from build123d import *

# Parameters (mm, degrees)
SKETCH_W      = 800
SKETCH_H      = 500
PAD_DEPTH     = 750
SKETCH001_W   = 816.672542
SKETCH001_H   = 515.040198
PAD001_DEPTH  = 50
SKETCH002_W   = 715.631729
SKETCH002_H   = 638.12648
POCKET_DEPTH  = 20
SKETCH003_R   = 15.413666
SKETCH003_R_2 = 14.535816
PAD002_DEPTH  = 10
SKETCH004_W   = 32.008468
SKETCH004_H   = 201.831192
PAD003_DEPTH  = 10


with BuildPart() as part:
    # Sketch → Pad (new body)
    with BuildSketch(Plane.XZ):
        with Locations((400, 250)):
            Rectangle(SKETCH_W, SKETCH_H)
    extrude(amount=PAD_DEPTH)

    # Sketch001 (on Face5 of Pad) → Pad001 (join)
    with BuildSketch(Plane(origin=(0, 0, 0), x_dir=(1, 0, 0), z_dir=(0, 1, 0))):
        with Locations((397.221163, -247.606335)):
            Rectangle(SKETCH001_W, SKETCH001_H)
    extrude(amount=-PAD001_DEPTH)

    # Sketch002 (on Face6 of Pad001) → Pocket (cut)
    with BuildSketch(Plane(origin=(0, 0, 0), x_dir=(1, 0, 0), z_dir=(0, 0, -1))):
        with Locations((402.8294, 386.143486)):
            Rectangle(SKETCH002_W, SKETCH002_H)
    extrude(amount=-POCKET_DEPTH, mode=Mode.SUBTRACT)

    # Sketch003 (on Face16 of Pocket) → Pad002 (join)
    with BuildSketch(Plane(origin=(0, 0, 20), x_dir=(1, 0, 0), z_dir=(0, 0, -1))):
        with Locations((80.433578, 384.418488)):
            Circle(SKETCH003_R)
        with Locations((79.198502, 264.994965)):
            Circle(SKETCH003_R_2)
    extrude(amount=PAD002_DEPTH)

    # Sketch004 (on Face20 of Pad002) → Pad003 (join)
    with BuildSketch(Plane(origin=(0, 0, 10), x_dir=(1, 0, 0), z_dir=(0, 0, -1))):
        with Locations((80.688408, 324.975487)):
            Rectangle(SKETCH004_W, SKETCH004_H)
    extrude(amount=PAD003_DEPTH)


solid = part.part
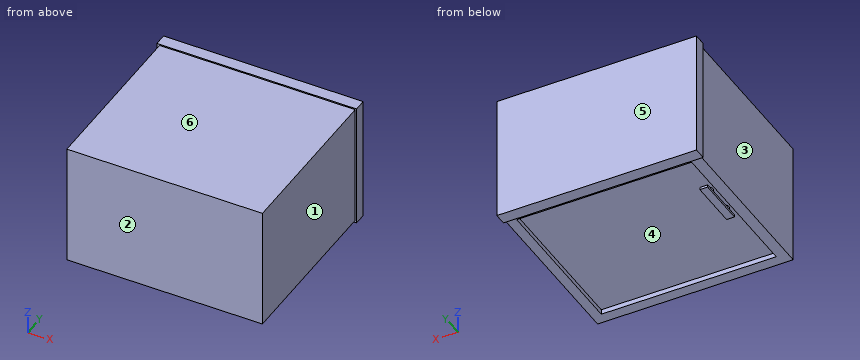
Here's how the part is built. I have some questions about the finished solid (model axes, mm). Face numbers are marked on the shaded views. A direction names the side the tool comes from. Round coordinates to 2 decimals unless told otherwise and drop trailing zeros. Loops run counter-clockwise (first coordinate to the right, second up) from the corner with the lowest first, then second, coordinate; pieces in that order, holes last. Notation, with made-up numbers: M -11,5.25 L 48,5.25 A31 ccw 48,29.25 Z; hole C 64,66.5 d1. An arc over 180 degrees is marked long. Write each question's results on one line, items separated by ' | '. Start each with the question number.
(1) On a 3-axis mill with a long thin cutter (end or side, diameter ignored), from which of +Z, -Z, +X, -X, +Y, -Y can I reach the whole of each face in a straight line? I mean the marked faces 1, 2 and 3. Say none if no direction works.
(2) Will these pins go through, and if not, where does the flat tip stop? P1, Ø2, axis at x = 563.5, y = -77, coming from the +Z side; P2, Ø5, axis at y = -286, z = 4.5, coming from the +X side; P3, Ø22, axis at y = -416.5, z = 10.5, coming from the -X side.
(3) Thinking about a two-plate mould opening in Y: for the marked faces 4, 5 and 6, which applies, pulls with the +Y half, pulls with the -Y half, needs draft (parallel to the pull), parting line crosses it, or undercut?
(4) I want a section at A-A (x = 120). Please give me the cut outline in (y, z), then the cut area to 3 significant figures.
(5) I want a section at C-C (y = -191.5). Please give me the cut outline in (x, z), then the cut area to 3 significant figures.
(6) I want a section at B-B (z = 350). Please give me the cut outline in (x, y).
(7) If I drill on probe 1 along X at (y, z) = (-676.5, 15); probe 2 along X at (y, z) = (-493.5, 214.5); probe 3 along Z at (x, y) = (150, -135.5), over which ranges is the centre line in solid material (lowest first)? Write a range as from..to.
Solved:
1) face 1: +Z, -Z, +X, -Y | face 2: +Z, -Z, +X, -X, -Y | face 3: +Z, -Z, -X, -Y
2) P1: stops at z = 500 | P2: stops at x = 800 | P3: stops at x = 0
3) face 4: undercut | face 5: pulls with the +Y half | face 6: needs draft
4) outline: M -750,0 L -705.21,0 L -705.21,20 L -67.08,20 L -67.08,0 L -50,0 L -50,-9.91 L 0,-9.91 L 0,505.13 L -50,505.13 L -50,500 L -750,500 Z | area: 363,000 mm²
5) outline: M 0,0 L 45.01,0 L 45.01,20 L 760.65,20 L 760.65,0 L 800,0 L 800,500 L 0,500 Z | area: 386,000 mm²
6) outline: M -11.12,-50 L 0,-50 L 0,-750 L 800,-750 L 800,-50 L 805.56,-50 L 805.56,0 L -11.12,0 Z
7) probe 1: x = 0..45.01, 760.65..800 | probe 2: x = 0..800 | probe 3: z = 20..500
